Could you check a few things on this model? Use its own coordinates, in mm. A direction names the side the tool comes from. Give positions to 0.01 mm unless a question says otherwise; leave off trailing zeros. Write each loop counter-clockwise with the first axis right and the second up, starting at its lowest first coordinate (ties: lowest second). Pieces come first, ordered by that corner, then holes. Notation, with made-up numbers: (-11.75, 85.5) -> (11.25, 85.5) arc R18 ccw to (11.25, 97.5) -> close; hole circle Ø9 at (-19.5, -35.5). An arc over 180 degrees is marked (long way). Write item = value, one per line. Start each with the question number.
```python
from build123d import *

# Parameters (mm, degrees)
SKETCH1_W           = 410
SKETCH1_H           = 76.2
SKETCH1_R           = 12.75
SKETCH1_R_2         = 6.125
BOSS_EXTRUDE1_DEPTH = 12.7
SKETCH2_R           = 6
CUT_EXTRUDE1_DEPTH  = 15
SKETCH4_OUTSIDE_W   = 495.558
SKETCH4_OUTSIDE_H   = 110.958
SKETCH4_OUTSIDE_W_2 = 410
SKETCH4_OUTSIDE_H_2 = 19
CUT_EXTRUDE2_DEPTH  = 30
M8_TAPPED_HOLE1_D   = 6.8


with BuildPart() as part:
    # Sketch1 → Boss-Extrude1 (new body, symmetric)
    with BuildSketch(Plane.XY):
        Rectangle(SKETCH1_W, SKETCH1_H)
        with Locations((0, 20.1)):
            Circle(SKETCH1_R, mode=Mode.SUBTRACT)
        with Locations((190, -27.9)):
            Circle(SKETCH1_R_2, mode=Mode.SUBTRACT)
        with Locations((-190, -27.9)):
            Circle(SKETCH1_R_2, mode=Mode.SUBTRACT)
    extrude(amount=BOSS_EXTRUDE1_DEPTH, both=True)

    # Sketch2 → Cut-Extrude1 (cut)
    with BuildSketch(Plane.XZ.offset(38.1)):
        Circle(SKETCH2_R)
        with Locations((-165, 0)):
            Circle(SKETCH2_R)
        with Locations((165, 0)):
            Circle(SKETCH2_R)
    extrude(amount=-CUT_EXTRUDE1_DEPTH, mode=Mode.SUBTRACT)

    # Sketch4 outside → Cut-Extrude2 (cut)
    with BuildSketch(Plane.XZ.offset(38.1)):
        Rectangle(SKETCH4_OUTSIDE_W, SKETCH4_OUTSIDE_H)
        Rectangle(SKETCH4_OUTSIDE_W_2, SKETCH4_OUTSIDE_H_2, mode=Mode.SUBTRACT)
    extrude(amount=-CUT_EXTRUDE2_DEPTH, mode=Mode.SUBTRACT)

    # M8 Tapped Hole1 (through all)
    with Locations(Plane.XY.offset(12.7)):
        with Locations((-60, 3.9), (-40, 3.9), (40, 3.9), (60, 3.9)):
            Hole(M8_TAPPED_HOLE1_D / 2)


solid = part.part
```
(1) I'm going to push flat-ended pins straight in: pin 1 (2.5 mm diameter, centred on x = -86.5, z = -11, fed in from -Y); pin 2 (3.5 mm diameter, centred on x = 167, z = 3, fed in from -Y); pin 3 (8 mm diameter, centred on x = -60, y = 3.9, fed in from -Z); pin 4 (24 mm diameter, centred on x = 22.5, y = -22, fed in from -Z). Where does each tip first touch, or does it pass through?
(2) If I drill on line 1 along Y through (x, z) = (-40, 4.25); line 2 along Y through (x, z) = (190, 4) (3 decimals); line 3 along Z through (x, y) = (-165, -26.5), over which ranges is the centre line in solid material (lowest first)? Write a range as from..to.
(3) Imagine slicing it at B-B (y = -27.9). Please give me the cut outline in (x, z) (3 decimals).
(4) Imagine slicing it at C-C (y = 25.5). Please give me the cut outline in (x, z).
(5) Imagine slicing it at D-D (z = 0). Please give me the cut outline in (x, y) (3 decimals), then the cut area to 3 significant figures.
(6) Imagine slicing it at A-A (x = 0). Please give me the cut outline in (y, z), then the cut area to 3 significant figures.
(7) On a 3-axis mill with a long thin cutter (end or side, diameter ignored), from which of +Z, -Z, +X, -X, +Y, -Y can I reach the whole of each face in a straight line? I mean faces 1 (the flat face through (-205, -1, 0)), 2 (the flat face through (0, -23.1, 0)), 3 (the flat face through (-3, -23, 9.5)). Say none if no direction works.
(8) We'd pull the mould along Y, two halves only. Please class faces 4 (the flat face through (-165, -23.1, 0)), 5 (the flat face through (-3, -23, -9.5)), 6 (the cylindrical face through (36.86, 2.6, -0.18)): released by +Y, released by -Y, zero draft, split by the parting line, or undercut.
Answers below:
q1.pin_1 = -8.1
q1.pin_2 = -23.1
q1.pin_3 = -12.7
q1.pin_4 = -9.5
q2.line_1 = -38.1..0.5, 7.3..38.1
q2.line_2 = -38.1..-34.025, -21.775..38.1
q2.line_3 = -9.5..-6, 6..9.5
q3.outline = (-205, -9.5) -> (-196.125, -9.5) -> (-196.125, 9.5) -> (-205, 9.5) -> close; (-183.875, -9.5) -> (183.875, -9.5) -> (183.875, 9.5) -> (-183.875, 9.5) -> close; (196.125, -9.5) -> (205, -9.5) -> (205, 9.5) -> (196.125, 9.5) -> close; hole circle Ø12 at (-165, 0); hole circle Ø12 at (0, 0); hole circle Ø12 at (165, 0)
q4.outline = (-205, -12.7) -> (-11.55, -12.7) -> (-11.55, 12.7) -> (-205, 12.7) -> close; (11.55, -12.7) -> (205, -12.7) -> (205, 12.7) -> (11.55, 12.7) -> close
q5.outline = (-205, -38.1) -> (-171, -38.1) -> (-171, -23.1) -> (-159, -23.1) -> (-159, -38.1) -> (-6, -38.1) -> (-6, -23.1) -> (6, -23.1) -> (6, -38.1) -> (159, -38.1) -> (159, -23.1) -> (171, -23.1) -> (171, -38.1) -> (205, -38.1) -> (205, 38.1) -> (-205, 38.1) -> close; hole circle Ø12.25 at (-190, -27.9); hole circle Ø6.8 at (-60, 3.9); hole circle Ø6.8 at (-40, 3.9); hole circle Ø25.5 at (0, 20.1); hole circle Ø6.8 at (40, 3.9); hole circle Ø6.8 at (60, 3.9); hole circle Ø12.25 at (190, -27.9)
q5.area = 29,800 mm^2
q6.outline = (-38.1, -9.5) -> (-8.1, -9.5) -> (-8.1, -12.7) -> (7.35, -12.7) -> (7.35, 12.7) -> (-8.1, 12.7) -> (-8.1, 9.5) -> (-38.1, 9.5) -> (-38.1, 6) -> (-23.1, 6) -> (-23.1, -6) -> (-38.1, -6) -> close; (32.85, -12.7) -> (38.1, -12.7) -> (38.1, 12.7) -> (32.85, 12.7) -> close
q6.area = 916 mm^2
q7.face_1 = +Z, -Z, -X, +Y, -Y
q7.face_2 = -Y
q7.face_3 = +Z, +X, -X, -Y
q8.face_4 = released by -Y
q8.face_5 = zero draft
q8.face_6 = undercut
